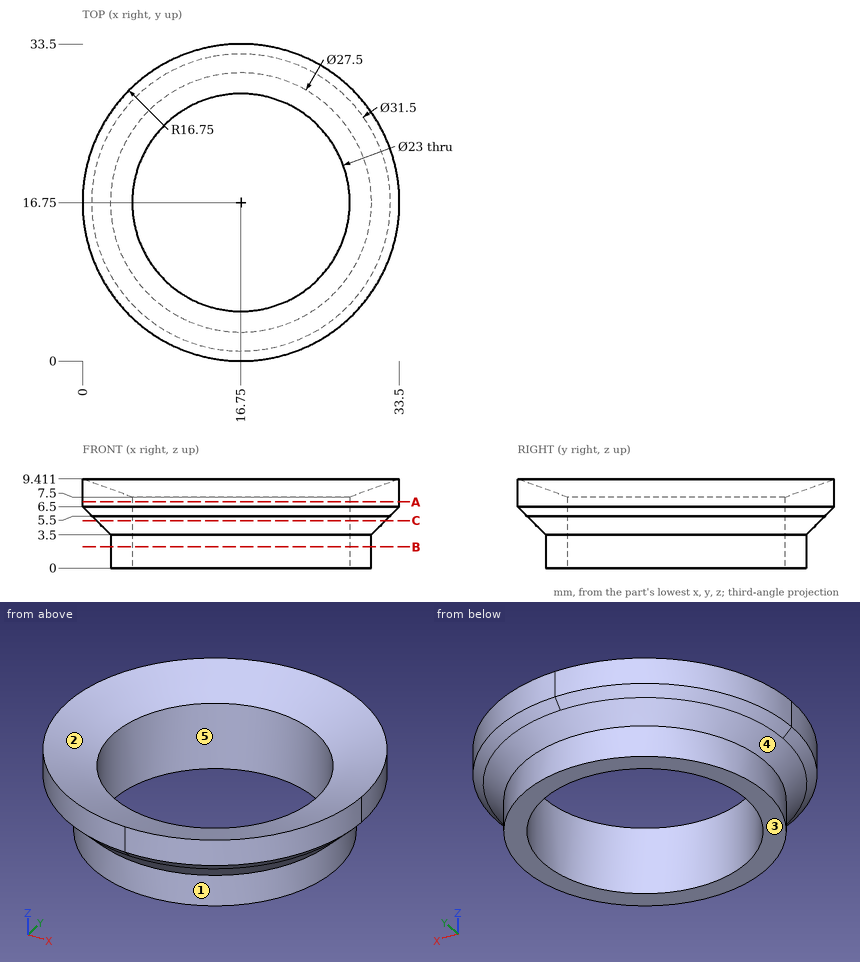
Here's the drawing with two shaded views (mm, measured from the low corner). I have some questions. A direction names the side the tool comes from. Coordinates: 2 decimals unless noted, no trailing zeros. Order: outer loops, then holes, each group sorted by start corner. A loop starts at its lowest first (then second) coordinate and runs counter-clockwise, first axis right, second up. Notation, with made-up numbers: (-12, 26) - (4, 26) arc R31 ccw to (4, 62) - close; hole circle Ø9 at (23.25, 85.5). An arc over 180 degrees is marked (long way). Answer in a Markdown table with one row per item. Add a question column.
(1) If we mould it in two halves opening along X, with no side actions, what happens to the marked faces 3, 4 and 5? For each: released by +X, released by -X, zero draft, split by the parting line, or undercut.
(2) Will these pins go through, and if not, where does the flat tip stop? pin 1 (4 mm diameter, centred on x = 4.5, y = 24, fed in from +Z); pin 2 (2 mm diameter, centred on x = 25, z = 7, fed in from +Y); pin 3 (5 mm diameter, centred on x = 20, z = 6.5, fed in from +Y); pin 4 (12 mm diameter, centred on x = 15, y = 19, fed in from +Z).
(3) If we section it at C-C, the plane z = 5: Please give me the cut outline in (x, y).
(4) If we section it at B-B, the plane z = 2.25: Please give me the cut outline in (x, y).
(5) I need wall thicknesses on L1, parallel to Y at x = 16.75, z = 2; L2, parallel to X at y = 15, z = 1.75; L3, parallel to Y at x = 16.75, z = 4. Which ranges of each line are inside material? Lowest first, please.
(6) If we section it at A-A, the plane z = 7: Please give me the cut outline in (x, y), then the cut area to 3 significant figures.
(7) On a 3-axis mill with a long thin cutter (end or side, diameter ignored), from which of +Z, -Z, +X, -X, +Y, -Y can I reach the whole of each face in a straight line? I mean the marked faces 1 and 2. Say none if no direction works.
Results are:
| question | item | result |
|---|---|---|
| 1 | face 3 | zero draft |
| 1 | face 4 | split by the parting line |
| 1 | face 5 | undercut |
| 2 | pin 1 | stops at z = 9.22 |
| 2 | pin 2 | stops at y = 31.85 |
| 2 | pin 3 | stops at y = 33.48 |
| 2 | pin 4 | passes through |
| 3 | outline | circle Ø30.5 at (16.75, 16.75); hole circle Ø23 at (16.75, 16.75) |
| 4 | outline | circle Ø27.5 at (16.75, 16.75); hole circle Ø23 at (16.75, 16.75) |
| 5 | L1 | y = 3 to 5.25, 28.25 to 30.5 |
| 5 | L2 | x = 3.11 to 5.38, 28.12 to 30.39 |
| 5 | L3 | y = 2.5 to 5.25, 28.25 to 31 |
| 6 | outline | circle Ø33.5 at (16.75, 16.75); hole circle Ø23 at (16.75, 16.75) |
| 6 | area | 466 mm2 |
| 7 | face 1 | -Z |
| 7 | face 2 | +Z |
